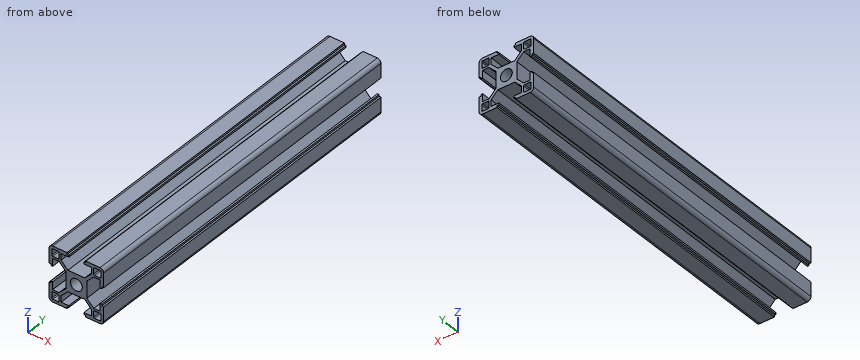
from build123d import *

# Parameters (mm, degrees)
SKETCH1_W           = 4
SKETCH1_H           = 4
SKETCH1_R           = 3.25
BOSS_EXTRUDE1_DEPTH = 196
SKETCH2_W           = 1
SKETCH2_H           = 1
CUT_EXTRUDE1_DEPTH  = 198.144616969
FILLET1_R           = 0.5


with BuildPart() as part:
    # Sketch1 → Boss-Extrude1 (new body)
    with BuildSketch(Plane(origin=(0, 0, 0), x_dir=(1, 0, 0), z_dir=(0, 1, 0))):
        with BuildLine():
            Line((-8.375, 9.50637085), (-8.375, 13))
            Line((-8.375, 13), (-4.125, 13))
            Line((-4.125, 13), (-4.125, 15))
            Line((-4.125, 15), (-13, 15))
            ThreePointArc((-13, 15), (-14.414213562, 14.414213562), (-15, 13))
            Line((-15, 13), (-15, 4.125))
            Line((-15, 4.125), (-13, 4.125))
            Line((-13, 4.125), (-13, 8.375))
            Line((-13, 8.375), (-9.50637085, 8.375))
            Line((-9.50637085, 8.375), (-5.75, 4.61862915))
            Line((-5.75, 4.61862915), (-5.75, -4.61862915))
            Line((-5.75, -4.61862915), (-9.50637085, -8.375))
            Line((-9.50637085, -8.375), (-13, -8.375))
            Line((-13, -8.375), (-13, -4.125))
            Line((-13, -4.125), (-15, -4.125))
            Line((-15, -4.125), (-15, -13))
            ThreePointArc((-15, -13), (-14.414213562, -14.414213562), (-13, -15))
            Line((-13, -15), (-4.125, -15))
            Line((-4.125, -15), (-4.125, -13))
            Line((-4.125, -13), (-8.375, -13))
            Line((-8.375, -13), (-8.375, -9.50637085))
            Line((-8.375, -9.50637085), (-4.61862915, -5.75))
            Line((-4.61862915, -5.75), (4.61862915, -5.75))
            Line((4.61862915, -5.75), (8.375, -9.50637085))
            Line((8.375, -9.50637085), (8.375, -13))
            Line((8.375, -13), (4.125, -13))
            Line((4.125, -13), (4.125, -15))
            Line((4.125, -15), (13, -15))
            ThreePointArc((13, -15), (14.414213562, -14.414213562), (15, -13))
            Line((15, -13), (15, -4.125))
            Line((15, -4.125), (13, -4.125))
            Line((13, -4.125), (13, -8.375))
            Line((13, -8.375), (9.50637085, -8.375))
            Line((9.50637085, -8.375), (5.75, -4.61862915))
            Line((5.75, -4.61862915), (5.75, 4.61862915))
            Line((5.75, 4.61862915), (9.50637085, 8.375))
            Line((9.50637085, 8.375), (13, 8.375))
            Line((13, 8.375), (13, 4.125))
            Line((13, 4.125), (15, 4.125))
            Line((15, 4.125), (15, 13))
            ThreePointArc((15, 13), (14.414213562, 14.414213562), (13, 15))
            Line((13, 15), (4.125, 15))
            Line((4.125, 15), (4.125, 13))
            Line((4.125, 13), (8.375, 13))
            Line((8.375, 13), (8.375, 9.50637085))
            Line((8.375, 9.50637085), (4.61862915, 5.75))
            Line((4.61862915, 5.75), (-4.61862915, 5.75))
            Line((-4.61862915, 5.75), (-8.375, 9.50637085))
        make_face()
        with Locations((-11.5, -11.5)):
            Rectangle(SKETCH1_W, SKETCH1_H, mode=Mode.SUBTRACT)
        with Locations((11.5, -11.5)):
            Rectangle(SKETCH1_W, SKETCH1_H, mode=Mode.SUBTRACT)
        Polygon((-9.5, 9.5), (-10.63137085, 9.5), (-13.5, 9.5), (-13.5, 13.5), (-9.5, 13.5), align=None, mode=Mode.SUBTRACT)
        with Locations(Location((0, 0, 0), (0, 0, 270))):
            Circle(SKETCH1_R, mode=Mode.SUBTRACT)
        with Locations((11.5, 11.5)):
            Rectangle(SKETCH1_W, SKETCH1_H, mode=Mode.SUBTRACT)
    extrude(amount=BOSS_EXTRUDE1_DEPTH)

    # Sketch2 → Cut-Extrude1 (cut, through all)
    with BuildSketch(Plane(origin=(0, 196, 0), x_dir=(1, 0, 0), z_dir=(0, 1, 0))):
        with Locations((14.5, 4.625)):
            Rectangle(SKETCH2_W, SKETCH2_H)
        with Locations((-4.625, 14.5)):
            Rectangle(SKETCH2_W, SKETCH2_H)
        with Locations((4.625, 14.5)):
            Rectangle(SKETCH2_W, SKETCH2_H)
        with Locations((14.5, -4.625)):
            Rectangle(SKETCH2_W, SKETCH2_H)
        with Locations((4.625, -14.5)):
            Rectangle(SKETCH2_W, SKETCH2_H)
        with Locations((-4.625, -14.5)):
            Rectangle(SKETCH2_W, SKETCH2_H)
        with Locations((-14.5, -4.625)):
            Rectangle(SKETCH2_W, SKETCH2_H)
        with Locations((-14.5, 4.625)):
            Rectangle(SKETCH2_W, SKETCH2_H)
    extrude(amount=-CUT_EXTRUDE1_DEPTH, mode=Mode.SUBTRACT)

    # Fillet1
    fillet1_edges = [part.edges().sort_by_distance(p)[0] for p in [
        (-9.5, 98, -13.5),
        (-13.5, 98, -13.5),
        (-13.5, 98, -9.5),
        (-9.5, 98, -9.5),
        (-9.5, 98, 9.5),
        (-13.5, 98, 9.5),
        (-13.5, 98, 13.5),
        (-9.5, 98, 13.5),
        (9.5, 98, -9.5),
        (13.5, 98, -9.5),
        (13.5, 98, -13.5),
        (9.5, 98, -13.5),
        (13.5, 98, 13.5),
        (13.5, 98, 9.5),
        (9.5, 98, 9.5),
        (9.5, 98, 13.5),
    ]]
    fillet(fillet1_edges, radius=FILLET1_R)


solid = part.part
Can you work these out from the model? Positions are in its coordinate system, mm. Coordinates: 2 decimals unless noted, no trailing zeros. Write each loop counter-clockwise with the first axis right and the second up, starting at its lowest first coordinate (ties: lowest second). Pieces come first, ordered by that corner, then holes. Notation, with made-up numbers: (32, -15) -> (71, -15) arc R21 ccw to (71, 21) -> close; hole circle Ø10 at (-10, 89.5). An arc over 180 degrees is marked (long way). Write item = value, one per line.
(1) For pin 1 (0.5 mm diameter, centred on y = 89.5, z = 4.5, fed in from -X); pin 2 (0.8 mm diameter, centred on y = 58, z = 14.5, fed in from -X); pin 3 (0.5 mm diameter, centred on y = 52, z = 4.5, fed in from +X), each with a flat end and sliding along its axis, tell me the tip position at first contact or that it passes through.
Verdict:
pin_1 = -14
pin_2 = -14.67
pin_3 = 14
(2) Imagine slicing it at C-C (y = 122.5). State how many separate pieces and enclosed holes the cut face has, and give its area (3 significant figures).
Verdict:
separate_pieces = 1
enclosed_holes = 5
area = 297 mm^2
(3) Imagine slicing it at B-B (x = 0). Please give me the cut outline in (y, z), and give its area (3 significant figures).
Verdict:
outline = (0, -5.75) -> (196, -5.75) -> (196, -3.25) -> (0, -3.25) -> close; (0, 3.25) -> (196, 3.25) -> (196, 5.75) -> (0, 5.75) -> close
area = 980 mm^2
(4) Imagine slicing it at A-A (z = 0). Please give me the cut outline in (x, y), and give its area (3 significant figures).
Verdict:
outline = (-5.75, 0) -> (-3.25, 0) -> (-3.25, 196) -> (-5.75, 196) -> close; (3.25, 0) -> (5.75, 0) -> (5.75, 196) -> (3.25, 196) -> close
area = 980 mm^2
(5) If I drill on probe 1 along X at (y, z) = (100.5, 4.25); probe 2 along X at (y, z) = (139, -6.5); probe 3 along X at (y, z) = (84, 0), over which ranges is the centre line in solid material (lowest first)?
Verdict:
probe_1 = -14 to -13, -5.75 to 5.75, 13 to 14
probe_2 = -15 to -13, -7.63 to -5.37, 5.37 to 7.63, 13 to 15
probe_3 = -5.75 to -3.25, 3.25 to 5.75
